```python
from build123d import *

# Parameters (mm, degrees)
F0_W     = 11
F0_H     = 14.5
F1_DEPTH = 26
F2_DEPTH = 26.5


with BuildPart() as f1:
    # F0 (on Top) → F1 (new body)
    with BuildSketch(Plane.XY):
        Polygon((37, 0), (0, 0), (0, -54), (37, -54), (37, -43.5), (37, -29), (13, -29), (13, -25), (37, -25), (37, -10.5), align=None)
        with Locations((42.5, -17.75)):
            Rectangle(F0_W, F0_H)
        with Locations((42.5, -36.25)):
            Rectangle(F0_W, F0_H)
    extrude(amount=F1_DEPTH)

    # F0 (on Top) → F2 (join)
    with BuildSketch(Plane.XY):
        Polygon((37, -27), (37, -25), (13, -25), (13, -29), (37, -29), align=None)
        Polygon((48, -25), (37, -25), (37, -27), (37, -29), (48, -29), align=None)
    extrude(amount=F2_DEPTH)


solid = f1.part
```
Could you check a few things on this model? Use its own coordinates, in mm. A direction names the side the tool comes from. Round coordinates to 2 decimals unless told otherwise and drop trailing zeros. Loops run counter-clockwise (first coordinate to the right, second up) from the corner with the lowest first, then second, coordinate; pieces in that order, holes last. Notation, with made-up numbers: (66, 80.5) - (113, 80.5) arc R10 ccw to (113, 96.5) - close; hole circle Ø3 at (29, 22.5). An arc over 180 degrees is marked (long way). Answer in a Markdown table with one row per item. Add a question column.
(1) I need wall thicknesses on line 1 along X through (y, z) = (-7.5, 13); line 2 along Z through (x, y) = (8, -12.5); line 3 along Y through (x, z) = (41.5, 6.5). Which ranges of each line are inside material? Lowest first, please.
(2) I'm going to push flat-ended pins straight in: pin 1 (8.5 mm diameter, centred on y = -5, z = 15, fed in from +X); pin 2 (9 mm diameter, centred on x = 44.5, z = 9, fed in from +Y); pin 3 (4 mm diameter, centred on x = 30, y = -8, fed in from +Z). Where does each tip first touch, or does it pass through?
(3) For faces 1 (the face through (42, -43.5, 13)), 2 (the face through (37, -5, 13)), 3 (the face through (19, 0, 13)), which set-ups out of +Z, -Z, +X, -X, +Y, -Y let a thin tool reach every point of the face, with its end or its side?
(4) If we section it at A-A (z = 9.75): Please give me the cut outline in (x, y), plus the area to 3 significant figures.
(5) If we section it at D-D (y = -4): Please give me the cut outline in (x, z).
(6) If we section it at B-B (x = 44.5): Please give me the cut outline in (y, z), plus the area to 3 significant figures.
(7) If we section it at C-C (y = -41): Please give me the cut outline in (x, z).
Model answer:
| question | item | result |
|---|---|---|
| 1 | line 1 | x = 0 to 37 |
| 1 | line 2 | z = 0 to 26 |
| 1 | line 3 | y = -43.5 to -10.5 |
| 2 | pin 1 | stops at x = 37 |
| 2 | pin 2 | stops at y = -10.5 |
| 2 | pin 3 | stops at z = 26 |
| 3 | face 1 | +Z, -Z, +X, -Y |
| 3 | face 2 | +Z, -Z, +X, +Y |
| 3 | face 3 | +Z, -Z, +X, -X, +Y |
| 4 | outline | (0, -54) - (37, -54) - (37, -43.5) - (48, -43.5) - (48, -10.5) - (37, -10.5) - (37, 0) - (0, 0) - close |
| 4 | area | 2,360 mm² |
| 5 | outline | (0, 0) - (37, 0) - (37, 26) - (0, 26) - close |
| 6 | outline | (-43.5, 0) - (-10.5, 0) - (-10.5, 26) - (-25, 26) - (-25, 26.5) - (-29, 26.5) - (-29, 26) - (-43.5, 26) - close |
| 6 | area | 860 mm² |
| 7 | outline | (0, 0) - (48, 0) - (48, 26) - (0, 26) - close |
